Check sheet for the modelled part. Datum: model origin and axes. Units: mm. A direction names the side the tool comes from. Give positions to 0.01 mm unless a question says otherwise; leave off trailing zeros. Loops run counter-clockwise (first coordinate to the right, second up) from the corner with the lowest first, then second, coordinate; pieces in that order, holes last. Notation, with made-up numbers: (19.5, -28.75) - (41.5, -28.75) arc R12 cw to (41.5, -18.75) - close; hole circle Ø6 at (-32.5, 27). An arc over 180 degrees is marked (long way). Use CSV: the item, a comma, the result in double quotes.
from build123d import *

# Parameters (mm, degrees)
SKETCH2_W           = 100
SKETCH2_H           = 100
BOSS_EXTRUDE1_DEPTH = 226.3
SHELL1_T            = -2
SKETCH3_W           = 83
SKETCH3_H           = 209.3
CUT_EXTRUDE1_DEPTH  = 253.411746953
SKETCH5_W           = 83
SKETCH5_H           = 209.3
CUT_EXTRUDE2_DEPTH  = 253.411746953
CHAMFER1_SIZE       = 0.5


with BuildPart() as part:
    # Sketch2 → Boss-Extrude1 (new body)
    with BuildSketch(Plane(origin=(0, 0, 0), x_dir=(1, 0, 0), z_dir=(0, 1, 0))):
        Rectangle(SKETCH2_W, SKETCH2_H)
    extrude(amount=BOSS_EXTRUDE1_DEPTH)

    # Shell1
    shell1_openings = [part.faces().sort_by_distance(p)[0] for p in [
        (0, 226.3, 0),
        (0, 0, 0),
    ]]
    offset(amount=SHELL1_T, openings=shell1_openings, kind=Kind.INTERSECTION)

    # Sketch3 → Cut-Extrude1 (cut, through all)
    with BuildSketch(Plane.XY.offset(50)):
        with Locations((0, 113.15)):
            Rectangle(SKETCH3_W, SKETCH3_H)
    extrude(amount=-CUT_EXTRUDE1_DEPTH, mode=Mode.SUBTRACT)

    # Sketch5 → Cut-Extrude2 (cut, through all)
    with BuildSketch(Plane(origin=(50, 0, 0), x_dir=(0, 0, -1), z_dir=(1, 0, 0))):
        with Locations((0, 113.15)):
            Rectangle(SKETCH5_W, SKETCH5_H)
    extrude(amount=-CUT_EXTRUDE2_DEPTH, mode=Mode.SUBTRACT)

    # Chamfer1
    chamfer1_edges = [part.edges().sort_by_distance(p)[0] for p in [
        (0, 226.3, 50),
        (48, 0, 0),
        (0, 0, -48),
        (48, 113.15, -48),
        (-48, 0, 0),
        (-48, 113.15, -48),
        (0, 0, 48),
        (-48, 113.15, 48),
        (48, 226.3, 0),
        (0, 226.3, -48),
        (-48, 226.3, 0),
        (0, 226.3, 48),
        (41.5, 113.15, -48),
        (0, 8.5, -48),
        (-41.5, 113.15, -48),
        (0, 217.8, -48),
        (41.5, 113.15, 50),
        (0, 217.8, 50),
        (-41.5, 113.15, 50),
        (0, 8.5, 50),
        (50, 226.3, 0),
        (0, 0, 50),
        (-48, 217.8, 0),
        (-48, 113.15, 41.5),
        (-48, 8.5, 0),
        (-48, 113.15, -41.5),
        (50, 0, 0),
        (50, 113.15, -41.5),
        (50, 217.8, 0),
        (50, 113.15, 41.5),
        (50, 8.5, 0),
        (50, 113.15, 50),
        (-50, 113.15, 50),
        (50, 113.15, -50),
    ]]
    chamfer(chamfer1_edges, length=CHAMFER1_SIZE)


solid = part.part
1. Sectioned sample at C-C, the plane y = 192. State how many separate pieces and enclosed holes the cut face has, and give its area (3 significant figures).
Completed:
separate pieces,"4"
enclosed holes,"0"
area,"119 mm²"
2. Set-up check for faces 1 (the face through (-48, 104.3, 42.4)), 2 (the face through (-44, 104, 50)): record each of +Z, -Z, +X, -X, +Y, -Y from which the full face is reachable in a straight line by a thin tool's end or side.
Completed:
face 1,"+Y, -Y"
face 2,"+Z, +X, -X, +Y, -Y"
3. Release check for a two-part mould opening along Z. For faces 3 (the face through (-45, 104, -50)), 4 (the face through (48, 104, 43)), 5 (the face through (50, 104, 44)) record: released by +Z, released by -Z, zero draft, split by the parting line, or undercut.
Completed:
face 3,"released by -Z"
face 4,"undercut"
face 5,"zero draft"
4. Sectioned sample at B-B, the plane z = 6. Record the boundary of the cut face in (x, y), and give its area (4 significant figures).
Completed:
outline,"(-50, 0) - (-48.5, 0) - (-48, 0.5) - (-48, 8) - (-48.5, 8.5) - (-50, 8.5) - close; (-50, 217.8) - (-48.5, 217.8) - (-48, 218.3) - (-48, 225.8) - (-48.5, 226.3) - (-50, 226.3) - close; (48, 0.5) - (48.5, 0) - (49.5, 0) - (50, 0.5) - (50, 8) - (49.5, 8.5) - (48, 8.5) - close; (48, 217.8) - (49.5, 217.8) - (50, 218.3) - (50, 225.8) - (49.5, 226.3) - (48.5, 226.3) - (48, 225.8) - close"
area,"66.75 mm²"
5. Scan line: line 1 along X through (y, z) = (190, 45). Record every from-to range of solid material in increasing order.
Completed:
line 1,"x = -50 to -48, 48 to 50"
6. Sectioned sample at A-A, the plane x = -15. Record the boundary of the cut face in (y, z), and give its area (4 significant figures).
Completed:
outline,"(0, -50) - (8.5, -50) - (8.5, -48.5) - (8, -48) - (0.5, -48) - (0, -48.5) - close; (0, 48.5) - (0.5, 48) - (8.5, 48) - (8.5, 49.5) - (8, 50) - (0.5, 50) - (0, 49.5) - close; (217.8, -50) - (226.3, -50) - (226.3, -48.5) - (225.8, -48) - (218.3, -48) - (217.8, -48.5) - close; (217.8, 48) - (225.8, 48) - (226.3, 48.5) - (226.3, 49.5) - (225.8, 50) - (218.3, 50) - (217.8, 49.5) - close"
area,"66.75 mm²"
